Input: part model. Units: mm. Frame: model coordinates. Face numbers are marked on the shaded views. A direction names the side the tool comes from. Give positions to 0.01 mm unless a question says otherwise; leave off trailing zeros. Write each loop counter-clockwise with the first axis right and the second up, starting at its lowest first coordinate (ties: lowest second). Pieces come first, ordered by that corner, then holes. Notation, with made-up numbers: (79, 32.25) -> (103, 32.25) arc R36 cw to (103, 71.25) -> close; hole circle Ø4 at (23, 10). An arc over 180 degrees is marked (long way). Answer as a JSON object with one key per item and string values. Group by question number.
from build123d import *

# Parameters (mm, degrees)
F0_W     = 59
F0_H     = 13
F1_DEPTH = 7
F2_R     = 6
F3_DEPTH = 3
F5_DEPTH = 70


with BuildPart() as f1:
    # F0 (on Top) → F1 (new body)
    with BuildSketch(Plane.XY):
        Rectangle(F0_W, F0_H)
    extrude(amount=F1_DEPTH)

    # F2 (on face) → F3 (cut)
    with BuildSketch(Plane.XY.offset(7)):
        with Locations((-20, 0)):
            Circle(F2_R)
        with Locations((20, 0)):
            Circle(F2_R)
    extrude(amount=-F3_DEPTH, mode=Mode.SUBTRACT)

    # F4 (on face) → F5 (cut)
    with BuildSketch(Plane.YZ.offset(29.5)):
        Polygon((2.194, 0), (6.5, 0), (6.5, 2.48607), align=None)
    extrude(amount=-F5_DEPTH, mode=Mode.SUBTRACT)


solid = f1.part
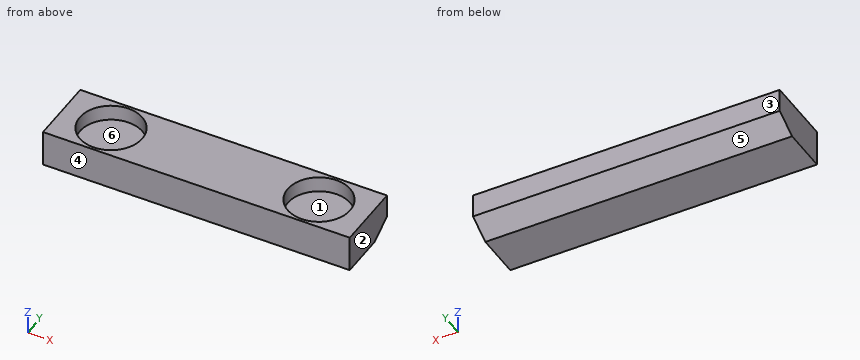
1. Line query: line 1 (X direction, y = -1.75, z = 5.75); line 2 (Y direction, x = -20, z = 5.1); line 3 (Z direction, x = 24, y = 0.25). Output: solid intervals per line, ascending.
2. Section A-A (x = 20). Return the cut outline in (y, z), plus the area to 3 significant figures.
3. Section D-D (x = 12.5). Return the cut outline in (y, z).
4. Reachability of the marked faces 5 and 6 from +Z, -Z, +X, -X, +Y, -Y: full face, straight path, thin tool, end or side. Return the list, or none.
5. Section B-B (y = 0). Return the cut outline in (x, z).
6. Section C-C (z = 5.75). Return the cut outline in (x, y).
7. Contact query for a flat-ended pin moving along its axis: pin 1 Ø2 at (x, y) = (19, 0.5) entering from +Z. Output: stop coordinate, or through.
8. Mould query, pull axis Y, two halves, no side actions, for the marked faces 1, 2, 3 and 4. Classes: pulls with the +Y half, pulls with the -Y half, needs draft (parallel to the pull), parting line crosses it, or undercut.
Working result:
{
 "1": {"line 1": "x = -29.5 to -25.74, -14.26 to 14.26, 25.74 to 29.5", "line 2": "y = -6.5 to -6, 6 to 6.5", "line 3": "z = 0 to 4"},
 "2": {"outline": "(-6.5, 0) -> (2.19, 0) -> (6.5, 2.49) -> (6.5, 7) -> (6, 7) -> (6, 4) -> (-6, 4) -> (-6, 7) -> (-6.5, 7) -> close", "area": "49.6 mm^2"},
 "3": {"outline": "(-6.5, 0) -> (2.19, 0) -> (6.5, 2.49) -> (6.5, 7) -> (-6.5, 7) -> close"},
 "4": {"face 5": "-Z, +X, -X, +Y", "face 6": "+Z"},
 "5": {"outline": "(-29.5, 0) -> (29.5, 0) -> (29.5, 7) -> (26, 7) -> (26, 4) -> (14, 4) -> (14, 7) -> (-14, 7) -> (-14, 4) -> (-26, 4) -> (-26, 7) -> (-29.5, 7) -> close"},
 "6": {"outline": "(-29.5, -6.5) -> (29.5, -6.5) -> (29.5, 6.5) -> (-29.5, 6.5) -> close; hole circle Ø12 at (-20, 0); hole circle Ø12 at (20, 0)"},
 "7": {"pin 1": "stops at z = 4"},
 "8": {"face 1": "undercut", "face 2": "needs draft", "face 3": "pulls with the +Y half", "face 4": "pulls with the -Y half"}
}
